Read the model definition and answer for the solid it produces. Units are mm, in the model's axes. Face numbers are marked on the shaded views. A direction names the side the tool comes from. Coordinates: 2 decimals unless noted, no trailing zeros. Write each loop counter-clockwise with the first axis right and the second up, starting at its lowest first coordinate (ties: lowest second). Pieces come first, ordered by that corner, then holes. Notation, with made-up numbers: (79, 38) - (121, 38) arc R26 cw to (121, 71) - close; hole circle Ø2 at (79, -2.75). An arc over 180 degrees is marked (long way). Return JSON: item names as keys, results as strings.
```python
from build123d import *

# Parameters (mm, degrees)
SKETCH1_W           = 20
SKETCH1_H           = 20
BOSS_EXTRUDE1_DEPTH = 4
SKETCH2_R           = 3.7
CUT_EXTRUDE1_DEPTH  = 2.6
SKETCH3_R           = 2.1
CUT_EXTRUDE2_DEPTH  = 29.403520909
SKETCH4_W           = 12
SKETCH4_H           = 4
BOSS_EXTRUDE2_DEPTH = 12
SKETCH7_W           = 20
SKETCH7_H           = 4
BOSS_EXTRUDE3_DEPTH = 10
SKETCH8_W           = 8
SKETCH8_H           = 20
BOSS_EXTRUDE4_DEPTH = 5
SKETCH9_W           = 8
SKETCH9_H           = 20
BOSS_EXTRUDE5_DEPTH = 5
SKETCH10_R          = 1.8
CUT_EXTRUDE5_DEPTH  = 42.243181255
SKETCH11_W          = 30
SKETCH11_H          = 30
CUT_EXTRUDE6_DEPTH  = 6
SKETCH12_R          = 1.45
CUT_EXTRUDE7_DEPTH  = 42.243181255
SKETCH13_W          = 8
SKETCH13_H          = 20
BOSS_EXTRUDE6_DEPTH = 2
SKETCH14_W          = 8
SKETCH14_H          = 20
BOSS_EXTRUDE7_DEPTH = 2
SKETCH15_W          = 16
SKETCH15_H          = 12
CUT_EXTRUDE8_DEPTH  = 39.845849199
FILLET2_R           = 3
FILLET4_R           = 2
FILLET5_START       = -21
FILLET5_DEPTH       = 22
FILLET6_R           = 3
FILLET7_R           = 1
FILLET8_R           = 1


with BuildPart() as part:
    # Sketch1 → Boss-Extrude1 (new body)
    with BuildSketch(Plane(origin=(0, 0, 0), x_dir=(0, 0, -1), z_dir=(1, 0, 0))):
        with Locations((-10, -10)):
            Rectangle(SKETCH1_W, SKETCH1_H)
    extrude(amount=BOSS_EXTRUDE1_DEPTH)

    # Sketch2 → Cut-Extrude1 (cut)
    with BuildSketch(Plane(origin=(4, 0, 0), x_dir=(0, 0, -1), z_dir=(1, 0, 0))):
        with Locations((-10, -10)):
            Circle(SKETCH2_R)
    extrude(amount=-CUT_EXTRUDE1_DEPTH, mode=Mode.SUBTRACT)

    # Sketch3 → Cut-Extrude2 (cut, through all)
    with BuildSketch(Plane(origin=(1.4, 0, 0), x_dir=(0, 0, -1), z_dir=(1, 0, 0))):
        with Locations((-10, -10)):
            Circle(SKETCH3_R)
    extrude(amount=-CUT_EXTRUDE2_DEPTH, mode=Mode.SUBTRACT)

    # Sketch4 → Boss-Extrude2 (add)
    with BuildSketch(Plane(origin=(4, 0, 0), x_dir=(0, 0, -1), z_dir=(1, 0, 0))):
        Polygon((-20, 0), (-20, -20), (-16, -20), (-16, -16), (-16, -4), (-16, 0), align=None)
        with Locations((-10, -18)):
            Rectangle(SKETCH4_W, SKETCH4_H)
        Polygon((-4, -16), (-4, -20), (0, -20), (0, -4), (-4, -4), align=None)
        Polygon((0, 0), (-16, 0), (-16, -4), (-4, -4), (0, -4), align=None)
    extrude(amount=BOSS_EXTRUDE2_DEPTH)

    # Sketch7 → Boss-Extrude3 (add)
    with BuildSketch(Plane(origin=(16, 0, 0), x_dir=(0, 0, -1), z_dir=(1, 0, 0))):
        with Locations((-10, -18)):
            Rectangle(SKETCH7_W, SKETCH7_H)
        with Locations((-10, -2)):
            Rectangle(SKETCH7_W, SKETCH7_H)
    extrude(amount=BOSS_EXTRUDE3_DEPTH)

    # Sketch8 → Boss-Extrude4 (add)
    with BuildSketch(Plane(origin=(0, -20, 0), x_dir=(-1, 0, 0), z_dir=(0, -1, 0))):
        with Locations((-22, -10)):
            Rectangle(SKETCH8_W, SKETCH8_H)
    extrude(amount=BOSS_EXTRUDE4_DEPTH)

    # Sketch9 → Boss-Extrude5 (add)
    with BuildSketch(Plane(origin=(0, 0, 0), x_dir=(1, 0, 0), z_dir=(0, 1, 0))):
        with Locations((22, -10)):
            Rectangle(SKETCH9_W, SKETCH9_H)
    extrude(amount=BOSS_EXTRUDE5_DEPTH)

    # Sketch10 → Cut-Extrude5 (cut, through all)
    with BuildSketch(Plane(origin=(0, 0, 0), x_dir=(-1, 0, 0), z_dir=(0, 0, -1))):
        with Locations(Location((-22, 1, 0), (0, 0, 90))):
            Circle(SKETCH10_R)
        with Locations(Location((-22, -21, 0), (0, 0, 90))):
            Circle(SKETCH10_R)
    extrude(amount=-CUT_EXTRUDE5_DEPTH, mode=Mode.SUBTRACT)

    # Sketch11 → Cut-Extrude6 (cut)
    with BuildSketch(Plane.ZY):
        with Locations((15, -5)):
            Rectangle(SKETCH11_W, SKETCH11_H)
    extrude(amount=-CUT_EXTRUDE6_DEPTH, mode=Mode.SUBTRACT)

    # Sketch12 → Cut-Extrude7 (cut, through all)
    with BuildSketch(Plane(origin=(0, 0, 0), x_dir=(1, 0, 0), z_dir=(0, 1, 0))):
        with Locations(Location((11, -10, 0), (0, 0, 270))):
            Circle(SKETCH12_R)
    extrude(amount=-CUT_EXTRUDE7_DEPTH, mode=Mode.SUBTRACT)

    # Sketch13 → Boss-Extrude6 (add)
    with BuildSketch(Plane.XY.offset(20)):
        with Locations((10, -10)):
            Rectangle(SKETCH13_W, SKETCH13_H)
    extrude(amount=BOSS_EXTRUDE6_DEPTH)

    # Sketch14 → Boss-Extrude7 (add)
    with BuildSketch(Plane(origin=(0, 0, 0), x_dir=(-1, 0, 0), z_dir=(0, 0, -1))):
        with Locations((-10, -10)):
            Rectangle(SKETCH14_W, SKETCH14_H)
    extrude(amount=BOSS_EXTRUDE7_DEPTH)

    # Sketch15 → Cut-Extrude8 (cut, through all)
    with BuildSketch(Plane.ZY.offset(-6)):
        with Locations((10, -10)):
            Rectangle(SKETCH15_W, SKETCH15_H)
    extrude(amount=-CUT_EXTRUDE8_DEPTH, mode=Mode.SUBTRACT)

    # Fillet2
    fillet2_edges = [part.edges().sort_by_distance(p)[0] for p in [
        (26, -16, 10),
        (26, -4, 10),
    ]]
    fillet(fillet2_edges, radius=FILLET2_R)

    # Fillet4
    fillet4_edges = [part.edges().sort_by_distance(p)[0] for p in [
        (26, -25, 10),
        (18, -25, 10),
        (26, 5, 10),
        (18, 5, 10),
    ]]
    fillet(fillet4_edges, radius=FILLET4_R)

    # Fillet5: read off the stored shape, not the designer's step
    # Fillet5 outline → Fillet5 (cut)
    with BuildSketch(Plane(origin=(0, 0, 0), x_dir=(1, 0, 0), z_dir=(0, 1, 0)).offset(FILLET5_START)):
        with BuildLine():
            Line((6, 2), (6, -2))
            ThreePointArc((6, -2), (7.171572875, 0.828427125), (10, 2))
            Line((10, 2), (6, 2))
        make_face()
        with BuildLine():
            ThreePointArc((10, -22), (7.171572875, -20.828427125), (6, -18))
            Line((6, -18), (6, -22))
            Line((6, -22), (10, -22))
        make_face()
    extrude(amount=FILLET5_DEPTH, mode=Mode.SUBTRACT)

    # Fillet6
    # the kernel refuses this fillet: 3 mm, written as the material it takes off along each edge
    with BuildSketch(Plane(origin=(14, -27.071067812, -2), x_dir=(-1, 0, 0), z_dir=(0, 1, 0))) as fillet6_piece_1:
        with BuildLine():
            CenterArc((2.828427125, 3), FILLET6_R, 199.471220634, 70.528779366)
            Line((0, 2), (-0.056568542, 1.98))
            ThreePointArc((-0.056568542, 1.98), (-0.06, 1), (-0.06, 0))
            Line((-0.06, 0), (0, -0.06))
            Line((0, -0.06), (2.828427125, -0.06))
            Line((2.828427125, -0.06), (2.828427125, 0))
        make_face()
    extrude(amount=34.142135624, mode=Mode.SUBTRACT)
    with BuildSketch(Plane(origin=(14, -27.071067812, 22), x_dir=(0, 0, -1), z_dir=(0, 1, 0))) as fillet6_piece_2:
        with BuildLine():
            CenterArc((3, 2.828427125), FILLET6_R, 180, 70.528779366)
            Line((0, 2.828427125), (-0.06, 2.828427125))
            Line((-0.06, 2.828427125), (-0.06, 0))
            Line((-0.06, 0), (0, -0.06))
            ThreePointArc((0, -0.06), (1, -0.06), (1.98, -0.056568542))
            Line((1.98, -0.056568542), (2, 0))
        make_face()
    extrude(amount=34.142135624, mode=Mode.SUBTRACT)

    # Fillet7
    fillet7_edges = [part.edges().sort_by_distance(p)[0] for p in [
        (18, -20, 10),
    ]]
    fillet(fillet7_edges, radius=FILLET7_R)

    # Fillet8
    fillet8_edges = [part.edges().sort_by_distance(p)[0] for p in [
        (18, 0, 10),
    ]]
    fillet(fillet8_edges, radius=FILLET8_R)


solid = part.part
```
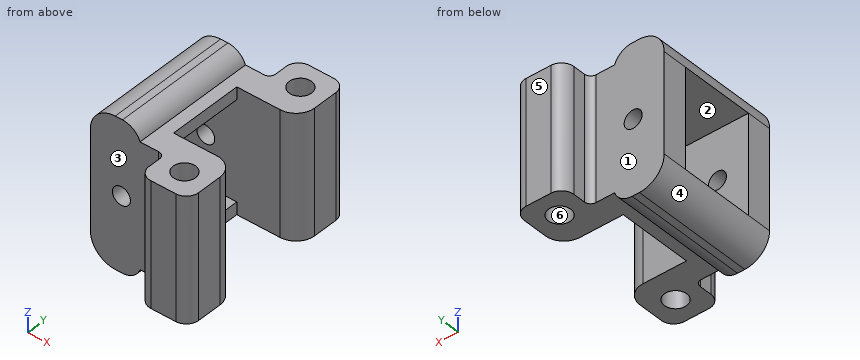
(1) Determine the mould class of the marked faces 4, 5 and 6 for opening direction X: +X half, -X half, draft (parallel to the pull), parting line (faces both ways), or undercut.
Answer:
{"face 4": "-X half", "face 5": "draft", "face 6": "undercut"}
(2) Which of the six approach directions +Z, -Z, +X, -X, +Y, -Y give full straight-line access (tool end or side, diameter ignored) to the marked faces 1, 2 and 3?
Answer:
{"face 1": "+Z, -Z, -X, +Y", "face 2": "+X, -X", "face 3": "+Z, -Z, -X, -Y"}
(3) A cutting plane is placed at D-D (y = -5.5). Determine the outline of the cut face in (x, z).
Answer:
{"outline": "(6, 2) arc R4 ccw to (10, -2) - (11.17, -2) arc R3 ccw to (14, 0) - (16, 0) - (16, 2) - close; (6, 18) - (16, 18) - (16, 20) - (14, 20) arc R3 ccw to (11.17, 22) - (10, 22) arc R4 ccw to start"}
(4) Flat-ended cylindrical pins translate along their axes: P1, Ø5.5, axis at x = 13.5, z = 6, coming from the -Y side; P2, Ø6, axis at x = 21, y = -5.5, coming from the -Z side; P3, Ø2, axis at y = -10, z = 1, coming from the +X side; P4, Ø3, axis at x = 22, y = -21, coming from the +Z side (3 decimals). Find the tip coordinate at first contact, or state that the pin passes through.
Answer:
{"P1": "y = -20", "P2": "z = 0", "P3": "x = 16", "P4": "through"}
(5) Straight lines are drawn through the part: line 1 (Y direction, x = 21.25, z = 4.25); line 2 (Z direction, x = 14.25, y = -14); line 3 (Y direction, x = 21.5, z = 19.75). For each, find the intervals that lie inside material, in ascending order. Write a range as from..to.
Answer:
{"line 1": "-25..-22.64, -19.36..-16, -4..-0.64, 2.64..5", "line 2": "0..2, 18..20", "line 3": "-25..-22.73, -19.27..-16, -4..-0.73, 2.73..5"}
(6) A cutting plane is placed at B-B (z = 10). State how many separate pieces and enclosed holes the cut face has, and give its area (3 significant figures).
Answer:
{"separate pieces": "4", "enclosed holes": "2", "area": "190 mm²"}
(7) A cutting plane is placed at C-C (z = 16.5). Determine the outline of the cut face in (x, y).
Answer:
{"outline": "(6, -20) - (17, -20) arc R1 cw to (18, -21) - (18, -23) arc R2 ccw to (20, -25) - (24, -25) arc R2 ccw to (26, -23) - (26, -19) arc R3 ccw to (23, -16) - (6, -16) - close; (6, -4) - (23, -4) arc R3 ccw to (26, -1) - (26, 3) arc R2 ccw to (24, 5) - (20, 5) arc R2 ccw to (18, 3) - (18, 1) arc R1 cw to (17, 0) - (6, 0) - close; hole circle Ø3.6 at (22, -21); hole circle Ø3.6 at (22, 1)"}
(8) A cutting plane is placed at A-A (x = 22). Determine the outline of the cut face in (y, z), and give its area (3 significant figures).
Answer:
{"outline": "(-25, 0) - (-22.8, 0) - (-22.8, 20) - (-25, 20) - close; (-19.2, 0) - (-16, 0) - (-16, 20) - (-19.2, 20) - close; (-4, 0) - (-0.8, 0) - (-0.8, 20) - (-4, 20) - close; (2.8, 0) - (5, 0) - (5, 20) - (2.8, 20) - close", "area": "216 mm²"}
